from build123d import *

# Parameters (mm, degrees)
ESQUISSE1_W                    = 36
ESQUISSE1_H                    = 36
BOSS_EXTRU_1_DEPTH             = 550
ENL_V_MAT_EXTRU_1_DEPTH        = 551.588775766
ENL_V_MAT_EXTRU_1_DEPTH_BACK   = 551.588775766
ESQUISSE2_W                    = 20
ESQUISSE2_H                    = 10
ESQUISSE3_R                    = 1.5
ENL_V_MAT_EXTRU_2_DEPTH        = 20
R_P_TITION_LIN_AIRE1_COUNT     = 11
R_P_TITION_LIN_AIRE1_PITCH     = 25
R_P_TITION_LIN_AIRE1_COL_COUNT = 11
R_P_TITION_LIN_AIRE1_COL_PITCH = 25


with BuildPart() as part:
    # Esquisse1 → Boss.-Extru.1 (new body)
    with BuildSketch(Plane.XY):
        Rectangle(ESQUISSE1_W, ESQUISSE1_H)
    extrude(amount=BOSS_EXTRU_1_DEPTH)

    # Esquisse2 → Enlèv. mat.-Extru.1 (cut, two sides: drawn at the far end of the back side and taken through both)
    with BuildSketch(Plane.XY.offset(550).offset(-ENL_V_MAT_EXTRU_1_DEPTH_BACK)):
        with Locations((8, 13)):
            Rectangle(ESQUISSE2_W, ESQUISSE2_H)
    extrude(amount=ENL_V_MAT_EXTRU_1_DEPTH + ENL_V_MAT_EXTRU_1_DEPTH_BACK, mode=Mode.SUBTRACT)

    # Esquisse3 → Enlèv. mat.-Extru.2 (cut)
    with BuildSketch(Plane(origin=(0, 8, 0), x_dir=(1, 0, 0), z_dir=(0, 1, 0))):
        with Locations(Location((8, -275, 0), (0, 0, 180))):
            Circle(ESQUISSE3_R)
    enl_v_mat_extru_2 = extrude(amount=-ENL_V_MAT_EXTRU_2_DEPTH, mode=Mode.SUBTRACT)

    # Répétition linéaire1: Enlèv. mat.-Extru.2 ×11
    with Locations(*[(0, 0, -i * R_P_TITION_LIN_AIRE1_PITCH) for i in range(1, R_P_TITION_LIN_AIRE1_COUNT)]):
        add(enl_v_mat_extru_2, mode=Mode.SUBTRACT)

    # Répétition linéaire1 col: Enlèv. mat.-Extru.2 ×11
    with Locations(*[(0, 0, i * R_P_TITION_LIN_AIRE1_COL_PITCH) for i in range(1, R_P_TITION_LIN_AIRE1_COL_COUNT)]):
        add(enl_v_mat_extru_2, mode=Mode.SUBTRACT)


solid = part.part
For this review, take the finished solid that the model builds, in its own axes (mm). A direction names the side the tool comes from. Coordinates: 2 decimals unless noted, no trailing zeros. Loops run counter-clockwise (first coordinate to the right, second up) from the corner with the lowest first, then second, coordinate; pieces in that order, holes last. Notation, with made-up numbers: (24, 32) -> (78, 32) arc R21 cw to (78, 38) -> close; hole circle Ø10 at (49, 17.25). An arc over 180 degrees is marked (long way). Write each question's results on one line, items separated by ' | '.
Q1. Add section A-A, the plane z = 116.5. State the section outline as (x, y) points.
Taken from the geometry:
outline: (-18, -18) -> (18, -18) -> (18, 8) -> (-2, 8) -> (-2, 18) -> (-18, 18) -> close
Q2. To check wall thickness, follow line 1 along X through (y, z) = (2, 250); line 2 along X through (y, z) = (12.5, 396.5); line 3 along Y through (x, z) = (10, 476). State the ranges of each line that lie inside material, in increasing order. Write a range as [from, to].
Taken from the geometry:
line 1: [-18, 6.5], [9.5, 18] | line 2: [-18, -2] | line 3: [-18, 8]
Q3. Machinability: for faces 1 (the flat face through (0, -18, 271)), 2 (the flat face through (-2, 13, 271)), which of the approach directions +Z, -Z, +X, -X, +Y, -Y give a long, thin tool a straight path to every point of the face, cutting with its end or side? Answer none if there is none.
Taken from the geometry:
face 1: +Z, -Z, +X, -X, -Y | face 2: +Z, -Z, +X, +Y
Q4. For pin 1 Ø1.8 at (x, z) = (8, 250) entering from +Y; pin 2 Ø3.5 at (x, z) = (8, 275) entering from +Y; pin 3 Ø1 at (y, z) = (10, 118) entering from +X, all flat-tipped, find the tip position at first contact; note any pin that passes through.
Taken from the geometry:
pin 1: y = -12 | pin 2: y = 8 | pin 3: x = -2
